```python
from build123d import *

# Parameters (mm, degrees)
EXTRUDE_4_DEPTH     = 20
EXTRUDE_5_DEPTH     = 80
CUT_EXTRUDE_2_DEPTH = 80
EXTRUDE_6_DEPTH     = 40


with BuildPart() as part:
    # 草圖1 → 填料-伸長4 (new body)
    with BuildSketch(Plane.XY):
        with BuildLine():
            Line((0.052876053, 14.999906804), (-29.946937555, 15.10565891))
            Line((-29.946937555, 15.10565891), (-55, 15.10565891))
            Line((-55, 15.10565891), (-55, 5.10565891))
            Line((-55, 5.10565891), (-75, 5.10565891))
            Line((-75, 5.10565891), (-75, -54.89434109))
            Line((-75, -54.89434109), (6.789733995, -13.37533223))
            ThreePointArc((6.789733995, -13.37533223), (14.5943097, 3.464985479), (0.052876053, 14.999906804))
        make_face()
    extrude(amount=EXTRUDE_4_DEPTH)

    # 草圖3 → 填料-伸長5 (add)
    with BuildSketch(Plane.XY):
        Polygon((-55, 15.10565891), (-85, 15.10565891), (-85, -54.89434109), (-75, -54.89434109), (-75, 5.10565891), (-55, 5.10565891), align=None)
    extrude(amount=EXTRUDE_5_DEPTH)

    # 草圖4 → 除料-伸長2 (cut)
    with BuildSketch(Plane(origin=(-75, 0, 0), x_dir=(0, 0, -1), z_dir=(1, 0, 0))):
        Polygon((-80, -24.89434109), (-50, -54.89434109), (-80, -54.89434109), align=None)
    extrude(amount=-CUT_EXTRUDE_2_DEPTH, mode=Mode.SUBTRACT)

    # 草圖5 → 填料-伸長6 (add)
    with BuildSketch(Plane.XY):
        with BuildLine():
            Line((-0.044063377, -9.999906804), (-30.044063377, -9.894154041))
            ThreePointArc((-30.044063377, -9.894154041), (-42.499922337, 2.649831673), (-29.955936623, 15.105690632))
            Line((-29.955936623, 15.105690632), (0.044063377, 14.999937869))
            ThreePointArc((0.044063377, 14.999937869), (12.499922337, 2.455952155), (-0.044063377, -9.999906804))
        make_face()
        with BuildLine():
            Line((-0.026438026, -4.999937869), (-30.026438026, -4.894185106))
            ThreePointArc((-30.026438026, -4.894185106), (-37.499953402, 2.632206322), (-29.973561974, 10.105721698))
            Line((-29.973561974, 10.105721698), (0.026438026, 9.999968935))
            ThreePointArc((0.026438026, 9.999968935), (7.499953402, 2.473577506), (-0.026438026, -4.999937869))
        make_face(mode=Mode.SUBTRACT)
    extrude(amount=EXTRUDE_6_DEPTH)


solid = part.part
```
CAD build for the part. Positions are in the model's coordinates, mm. A direction names the side the tool comes from. Coordinates: 2 decimals unless noted, no trailing zeros. Order: outer loops, then holes, each group sorted by start corner. A loop starts at its lowest first (then second) coordinate and runs counter-clockwise, first axis right, second up. Notation, with made-up numbers: M 31,-2 L 65,-2 A29 ccw 65,22 Z; hole C 1.5,48 d6. An arc over 180 degrees is marked long. Answer as CSV lines item,"result".
1) Flat gauge pins, fed straight in: P1, Ø10, axis at y = -3.5, z = 67, coming from the +X side; P2, Ø7.5, axis at x = -27, y = 6, coming from the +Z side; P3, Ø6, axis at y = 3, z = 42, coming from the +X side. Where does each tip first touch, or does it go through?
Verdict:
P1,"x = -75"
P2,"z = 20"
P3,"x = 12.5"
2) Cut at A-A (z = 27). List the corners of the cut face in (x, y).
Verdict:
outline,"M -85,-54.89 L -75,-54.89 L -75,5.11 L -55,5.11 L -55,15.11 L -85,15.11 Z; M -30.04,-9.89 L -0.04,-10 A12.5 ccw 0.04,15 L -29.96,15.11 A12.5 ccw Z; hole M -30.03,-4.89 L -0.03,-5 A7.5 ccw 0.03,10 L -29.97,10.11 A7.5 ccw Z"
3) Cut at B-B (z = 14). List the corners of the cut face in (x, y).
Verdict:
outline,"M -85,-54.89 L -75,-54.89 L 6.79,-13.38 A15 ccw 0.05,15 L -29.96,15.11 A12.5 ccw -30.05,15.11 L -85,15.11 Z"
4) Cut at C-C (x = -16.5). List the corners of the cut face in (y, z), then the cut area to 3 significant figures.
Verdict:
outline,"M -25.2,0 L 15.06,0 L 15.06,40 L 10.06,40 L 10.06,20 L -4.94,20 L -4.94,40 L -9.94,40 L -9.94,20 L -25.2,20 Z"
area,"1,010 mm2"
5) Drill centre lines: L1, parallel to Y at x = -3.5, z = 23.5; L2, parallel to Z at x = -44, y = 10; L3, parallel to Y at x = -56, z = 70. Where is each one in solid material? Low to high. Write a range as from..to.
Verdict:
L1,"-9.99..-4.99, 10.01..15.01"
L2,"0..20"
L3,"5.11..15.11"
6) Cut at D-D (y = -3.5). List the corners of the cut face in (x, z).
Verdict:
outline,"M -85,0 L 14.59,0 L 14.59,20 L 10.97,20 L 10.97,40 L 4.5,40 L 4.5,20 L -34.36,20 L -34.36,40 L -40.91,40 L -40.91,20 L -75,20 L -75,80 L -85,80 Z"
7) Mould opens along X. For faces 1 (the cylindrical face through (14.656, 3.192, 9.86)), 2 (the flat face through (-85, -19, 39)), 3 (the flat face through (-41, -19, 20)), 4 (the flat face through (-47, -12, 0)) say: released by +X, released by -X, zero draft, split by the parting line, or undercut.
Verdict:
face 1,"released by +X"
face 2,"released by -X"
face 3,"undercut"
face 4,"zero draft"
8) 3-axis set-ups, long thin cutter, end or side, ignore diameter. For faces 5 (the cylindrical face through (-37.5, 2.5, 29.9)), 6 (the flat face through (-55, 10, 50)), 7 (the flat face through (-65, 5.106, 50)), 8 (the flat face through (-15, -6, 40)): which of +Z, -Z, +X, -X, +Y, -Y reach the whole face in a straight line?
Verdict:
face 5,"+Z"
face 6,"+Z, +Y, -Y"
face 7,"+Z, -Y"
face 8,"+Z, +X, +Y, -Y"
